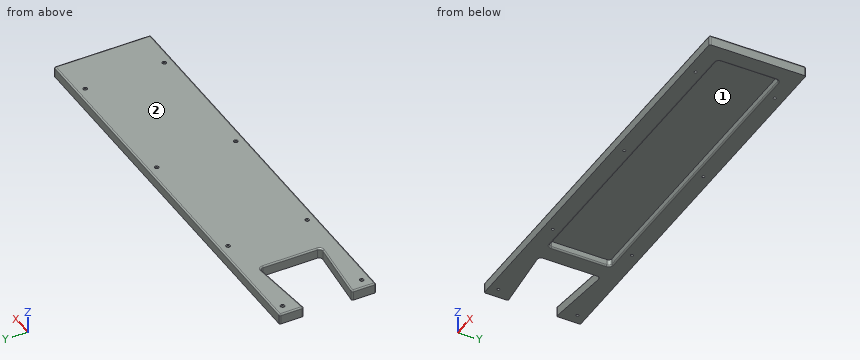
from build123d import *

# Parameters (mm, degrees)
F1_DEPTH       = 7.5
F3_DEPTH       = 10
F5_D           = 4
F5_CSINK_D     = 6
F5_CSINK_ANGLE = 90
F6_R           = 2


# Not quite as in the source:
# - a feature names something its author has since deleted; it is built from what else it names


with BuildPart() as f1:
    # F0 (on Top) → F1 (new body, symmetric)
    with BuildSketch(Plane.XY):
        with BuildLine():
            Line((-300, -70), (300, -70))
            Line((300, -70), (300, 70))
            Line((300, 70), (-300, 70))
            Line((-300, 70), (-300, 35))
            Line((-300, 35), (-205.4975185951, 44.4502481405))
            ThreePointArc((-205.4975185951, 44.4502481405), (-201.6449733962, 43.1823248572), (-200, 39.4750621894))
            Line((-200, 39.4750621894), (-200, 0))
            Line((-200, 0), (-200, -39.4750621894))
            ThreePointArc((-200, -39.4750621894), (-201.6449733962, -43.1823248572), (-205.4975185951, -44.4502481405))
            Line((-205.4975185951, -44.4502481405), (-300, -35))
            Line((-300, -35), (-300, -70))
        make_face()
    extrude(amount=F1_DEPTH, both=True)

    # F2 (on face) → F3 (cut)
    with BuildSketch(Plane(origin=(0, 0, -7.5), x_dir=(1, 0, 0), z_dir=(0, 0, -1))):
        with BuildLine():
            Line((-175, 40), (-175, 0))
            Line((-175, 0), (-175, -40))
            ThreePointArc((-175, -40), (-173.5355339059, -43.5355339059), (-170, -45))
            Line((-170, -45), (270, -45))
            ThreePointArc((270, -45), (273.5355339059, -43.5355339059), (275, -40))
            Line((275, -40), (275, 0))
            Line((275, 0), (275, 40))
            ThreePointArc((275, 40), (273.5355339059, 43.5355339059), (270, 45))
            Line((270, 45), (-170, 45))
            ThreePointArc((-170, 45), (-173.5355339059, 43.5355339059), (-175, 40))
        make_face()
    extrude(amount=-F3_DEPTH, mode=Mode.SUBTRACT)

    # F5 (through all)
    with Locations(Plane.XY.offset(7.5)):
        with Locations((-285, 57.5), (-285, -57.5), (-140, -57.5), (50, -57.5), (240, -57.5), (240, 57.5), (50, 57.5), (-140, 57.5)):
            CounterSinkHole(F5_D / 2, F5_CSINK_D / 2, counter_sink_angle=F5_CSINK_ANGLE)

    # F6
    f6_edges = [f1.edges().sort_by_distance(p)[0] for p in [
        (0, -70, 7.5),
        (-300, -52.5, 7.5),
        (-252.748759, -39.725124, 7.5),
        (0, 70, 7.5),
        (-300, 52.5, 7.5),
        (300, 0, 7.5),
        (-175, 0, -7.5),
        (-300, 35, 0),
        (-300, -70, 0),
        (-300, 70, 0),
        (300, 70, 0),
        (300, -70, 0),
        (-300, -35, 0),
    ]]
    fillet(f6_edges, radius=F6_R)


solid = f1.part
The listing builds one solid part. Answer for the finished solid, in the listing's coordinates (mm). Face numbers are marked on the shaded views. Give positions to 0.01 mm unless a question says otherwise; leave off trailing zeros. Write each loop counter-clockwise with the first axis right and the second up, starting at its lowest first coordinate (ties: lowest second). Pieces come first, ordered by that corner, then holes. Notation, with made-up numbers: (-33, 73.5) - (-25, 73.5) arc R14 ccw to (-25, 88.5) - close; hole circle Ø4 at (89.25, 54.5). An arc over 180 degrees is marked (long way). One line per question, with ' | ' between items. Start each with the question number.
1. Straight lines are drawn through the part: line 1 (X direction, y = -57.5, z = 0.25); line 2 (Y direction, x = 50, z = -1.75); line 3 (X direction, y = 57, z = 3.5). For each, find the intervals that lie inside material, in ascending order.
2. Given P1, Ø2, axis at x = 113, y = 24.5, coming from the -Z side; P2, Ø3, axis at x = -285, y = 57.5, coming from the +Z side; P3, Ø6.5, axis at x = -140, y = -57.5, coming from the +Z side; P4, Ø6.5, axis at y = 15.5, z = 2, coming from the -X side, each flat-ended and moving along its own axis, determine where each tip first touches the part or whether it passes through.
3. Section B-B, the plane x = -32.5 is taken. Determine the outline of the cut face in (y, z).
4. Determine the mould class of the marked faces 1 and 2 for opening direction X: +X half, -X half, draft (parallel to the pull), parting line (faces both ways), or undercut.
5. Section C-C, the plane y = 0 is taken. Determine the outline of the cut face in (x, z).
6. Section A-A, the plane z = -3.25 is taken. Count the separate pieces of the cut face and the enclosed holes in it, then the cut area to 3 significant figures.
Result:
1) line 1: x = -300 to -287, -283 to -142, -138 to 48, 52 to 238, 242 to 300 | line 2: y = -70 to -59.5, -55.5 to -45, 45 to 55.5, 59.5 to 70 | line 3: x = -300 to -286.94, -283.06 to -141.94, -138.06 to 48.06, 51.94 to 238.06, 241.94 to 300
2) P1: stops at z = 2.5 | P2: passes through | P3: stops at z = 7.5 | P4: stops at x = -200
3) outline: (-70, -7.5) - (-47, -7.5) arc R2 ccw to (-45, -5.5) - (-45, 2.5) - (45, 2.5) - (45, -5.5) arc R2 ccw to (47, -7.5) - (70, -7.5) - (70, 5.5) arc R2 ccw to (68, 7.5) - (-68, 7.5) arc R2 ccw to (-70, 5.5) - close
4) face 1: undercut | face 2: draft
5) outline: (-200, -7.5) - (-177, -7.5) arc R2 ccw to (-175, -5.5) - (-175, 2.5) - (275, 2.5) - (275, -5.5) arc R2 ccw to (277, -7.5) - (300, -7.5) - (300, 5.5) arc R2 ccw to (298, 7.5) - (-198, 7.5) arc R2 ccw to (-200, 5.5) - close
6) separate pieces: 1 | enclosed holes: 9 | area: 35,400 mm2
